For this review, take the finished solid that the model builds, in its own axes (mm). Face numbers are marked on the shaded views. Round coordinates to 2 decimals unless told otherwise and drop trailing zeros.
1) Mouldability with a two-part tool opening along Y and no side actions: class the marked faces 1 and 2 as pulls with the +Y half, pulls with the -Y half, needs draft (parallel to the pull), parting line crosses it, or undercut.
2) Wall thickness on L1, parallel to X at y = 110.5, z = 1.15; L2, parallel to X at y = 97.75, z = 1.4; L3, parallel to Y at x = 173.5, z = 1.5: over which ranges is each line inside the solid? List them lowest first.
3) Take a section at A-A (z = 0.85). Give the number of separate pieces and of enclosed holes in the cut face, then the cut area to 3 significant figures.
4) Insertion check: pin 1 (1 mm diameter, centred on x = 175.19, y = 108.29, fed in from -Z). The pin has a flat end and moves straight along its axis. Give the tip position at first contact, or say it passes through.
Autodesk Inventor part; units mm, degrees
ref_plane "BoardFrontPlane" through (0, 0, 0) normal (0, 0, 1) x (1, 0, 0)
ref_plane "YZ Plane" through (0, 0, 0) normal (1, 0, 0) x (0, 1, 0)
ref_plane "XZ Plane" through (0, 0, 0) normal (0, 1, 0) x (-1, 0, 0)
ref_plane "BoardFrontPlane" through (0, 0, 0) normal (0, 0, 1) x (1, 0, 0)
sketch "Sketch1" plane through (0, 0, 0) normal (0, 0, 1) x (1, 0, 0)
  line L0 (161.6857, 93.5857) -> (161.6857, 113.5857)
  line L1 (161.6857, 113.5857) -> (183.6857, 113.5857)
  line L2 (183.6857, 113.5857) -> (183.6857, 93.5857)
  line L3 (183.6857, 93.5857) -> (161.6857, 93.5857)
extrude "BoardOutline" add sketch "Sketch1" along normal blind 1.5954
sketch "Sketch10" plane through (0, 0, 1.5954) normal (0, 0, 1) x (1, 0, 0)
  point P0 (175.1857, 108.2857)
hole "CN3-1" at (175.1857, 108.2857, 1.5954) direction (0, 0, -1) diameter 1.6 end through all
sketch "Sketch11" plane through (0, 0, 1.5954) normal (0, 0, 1) x (1, 0, 0)
  point P0 (170.1857, 108.2857)
hole "CN3-2" at (170.1857, 108.2857, 1.5954) direction (0, 0, -1) diameter 1.6 end through all
sketch "Sketch12" plane through (0, 0, 1.5954) normal (0, 0, 1) x (1, 0, 0)
  point P0 (164.6857, 110.5857)
hole "Free-1" at (164.6857, 110.5857, 1.5954) direction (0, 0, -1) diameter 3.2 end through all
sketch "Sketch13" plane through (0, 0, 1.5954) normal (0, 0, 1) x (1, 0, 0)
  point P0 (180.6857, 96.5857)
hole "Free-0" at (180.6857, 96.5857, 1.5954) direction (0, 0, -1) diameter 3.2 end through all
sketch "img_Top" plane through (0, 0, 1.5954) normal (0, 0, 1) x (1, 0, 0)
  line L0 (161.6857, 113.5857) -> (183.6857, 113.5857) construction
  line L1 (183.6857, 113.5857) -> (183.6857, 93.5926) construction
  line L2 (183.6857, 93.5926) -> (161.6857, 93.5926) construction
  line L3 (161.6857, 93.5926) -> (161.6857, 113.5857) construction
decal "Decal_Top"
sketch "img_Bottom" plane through (0, 0, -1.5954) normal (0, 0, -1) x (1, 0, 0)
  line L0 (161.6857, -93.5857) -> (183.6857, -93.5857) construction
  line L1 (183.6857, -93.5857) -> (183.6857, -113.5787) construction
  line L2 (183.6857, -113.5787) -> (161.6857, -113.5787) construction
  line L3 (161.6857, -113.5787) -> (161.6857, -93.5857) construction
decal "Decal_Bottom"
sketch "Sketch16" plane through (0, 0, 1.5954) normal (0, 0, 1) x (1, 0, 0)
  point P0 (172.0857, 99.1607)
hole "CN2-4" at (172.0857, 99.1607, 1.5954) direction (0, 0, -1) diameter 0.6 end through all
sketch "Sketch17" plane through (0, 0, 1.5954) normal (0, 0, 1) x (1, 0, 0)
  point P0 (172.0857, 100.3607)
hole "CN2-1" at (172.0857, 100.3607, 1.5954) direction (0, 0, -1) diameter 0.6 end through all
sketch "Sketch18" plane through (0, 0, 1.5954) normal (0, 0, 1) x (1, 0, 0)
  point P0 (173.2857, 99.1607)
hole "CN2-3" at (173.2857, 99.1607, 1.5954) direction (0, 0, -1) diameter 0.6 end through all
sketch "Sketch19" plane through (0, 0, 1.5954) normal (0, 0, 1) x (1, 0, 0)
  point P0 (173.2857, 100.3607)
hole "CN2-2" at (173.2857, 100.3607, 1.5954) direction (0, 0, -1) diameter 0.6 end through all
sketch "Sketch20" plane through (0, 0, 1.5954) normal (0, 0, 1) x (1, 0, 0)
  point P0 (169.1857, 96.1607)
hole "CN2-0_SEOGABLU" at (169.1857, 96.1607, 1.5954) direction (0, 0, -1) diameter 1 end through all
sketch "Sketch21" plane through (0, 0, 1.5954) normal (0, 0, 1) x (1, 0, 0)
  point P0 (176.1857, 96.1607)
hole "CN2-0_AERYPNHJ" at (176.1857, 96.1607, 1.5954) direction (0, 0, -1) diameter 1 end through all
sketch "Sketch22" plane through (0, 0, 1.5954) normal (0, 0, 1) x (1, 0, 0)
  point P0 (172.6857, 97.6857)
hole "CN1-2" at (172.6857, 97.6857, 1.5954) direction (0, 0, -1) diameter 0.8 end through all
sketch "Sketch23" plane through (0, 0, 1.5954) normal (0, 0, 1) x (1, 0, 0)
  point P0 (170.1457, 97.6857)
hole "CN1-3" at (170.1457, 97.6857, 1.5954) direction (0, 0, -1) diameter 0.8 end through all
sketch "Sketch24" plane through (0, 0, 1.5954) normal (0, 0, 1) x (1, 0, 0)
  point P0 (175.2257, 97.6857)
hole "CN1-1" at (175.2257, 97.6857, 1.5954) direction (0, 0, -1) diameter 0.8 end through all
properties part number "valve_driver_BOARD"
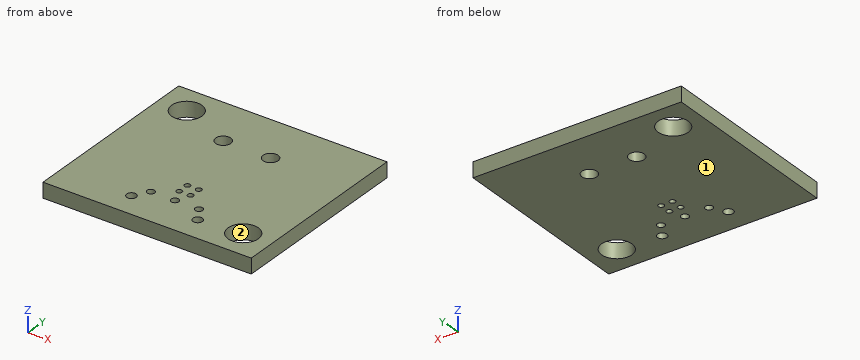
Response:
1. face 1: needs draft
1. face 2: undercut
2. L1: x = 161.69 to 163.09, 166.28 to 183.69
2. L2: x = 161.69 to 169.75, 170.54 to 172.29, 173.08 to 174.83, 175.62 to 179.59, 181.78 to 183.69
2. L3: y = 93.59 to 98.95, 99.37 to 100.15, 100.57 to 113.59
3. separate pieces: 1
3. enclosed holes: 13
3. area: 416 mm2
4. pin 1: passes through
